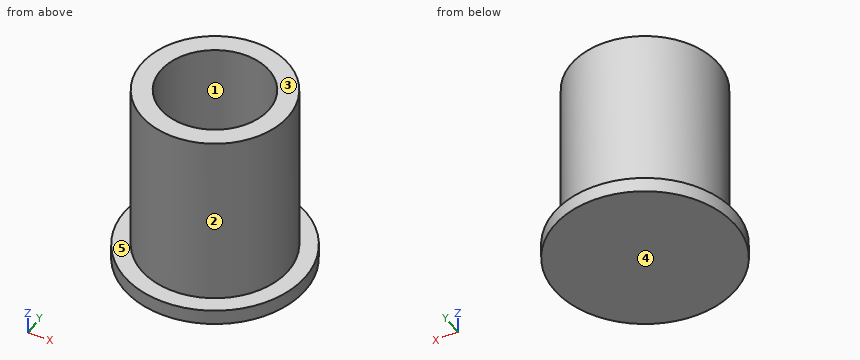
```python
from build123d import *

# Parameters (mm, degrees)
SKETCH_R     = 3
PAD_DEPTH    = 0.5
SKETCH001_R  = 2.435
PAD001_DEPTH = 5.8
SKETCH002_R  = 1.8
POCKET_DEPTH = 5.8


with BuildPart() as part:
    # Sketch (on Face1 of CopyBox) → Pad (new body)
    with BuildSketch(Plane.XY.offset(8)):
        Circle(SKETCH_R)
    extrude(amount=PAD_DEPTH)

    # Sketch001 (on Face3 of Pad) → Pad001 (join)
    with BuildSketch(Plane.XY.offset(8.5)):
        Circle(SKETCH001_R)
    extrude(amount=PAD001_DEPTH)

    # Sketch002 (on Face5 of Pad001) → Pocket (cut)
    with BuildSketch(Plane.XY.offset(14.3)):
        Circle(SKETCH002_R)
    extrude(amount=-POCKET_DEPTH, mode=Mode.SUBTRACT)


solid = part.part
```
Geometry check sheet. Reference: the model listing, model coordinates, mm. Face numbers are marked on the shaded views. A direction names the side the tool comes from. Round coordinates to 2 decimals unless told otherwise and drop trailing zeros. Loops run counter-clockwise (first coordinate to the right, second up) from the corner with the lowest first, then second, coordinate; pieces in that order, holes last. Notation, with made-up numbers: M -0.5,58.25 L 54.5,58.25 A19 cw 54.5,88.25 Z; hole C 5.5,60 d5. An arc over 180 degrees is marked long. Return JSON: item names as keys, results as strings. Group by question number.
(1) Scan lines: line 1 along Y through (x, z) = (0, 12.5) (3 decimals); line 2 along Z through (x, y) = (-1.25, -0.4); line 3 along X through (y, z) = (0.9, 11). Record each from-to range of solid material in increasing order. Write a range as [from, to].
(2) Section check B-B, the plane x = 0. Enter the section's corners in (y, z) (3 decimals).
(3) Section check D-D, the plane y = 2.35. Enter the section's corners in (x, z), and give its area (3 significant figures).
(4) Set-up check for the marked faces 4 and 5: record each of +Z, -Z, +X, -X, +Y, -Y from which the full face is reachable in a straight line by a thin tool's end or side.
(5) Section check A-A, the plane z = 11.25. Enter the section's corners in (x, y) (3 decimals).
(6) Mould release check, pull along X, two halves, no side actions. Record for the marked faces 1, 2 and 3: pulls with the +X half, pulls with the -X half, needs draft (parallel to the pull), parting line crosses it, or undercut.
(7) Go/stop test with flat-tipped pins: pin 1 (3 mm diameter, centred on y = 2, z = 10.5, fed in from +X); pin 2 (1.5 mm diameter, centred on x = -1, z = 13.5, fed in from -Y); pin 3 (1.8 mm diameter, centred on x = -0.5, y = -0.5, fed in from +Z). Record where each tip stops, or that it passes through.
Data:
{
 "1": {"line 1": "[-2.435, -1.8], [1.8, 2.435]", "line 2": "[8, 8.5]", "line 3": "[-2.26, -1.56], [1.56, 2.26]"},
 "2": {"outline": "M -3,8 L 3,8 L 3,8.5 L 2.435,8.5 L 2.435,14.3 L 1.8,14.3 L 1.8,8.5 L -1.8,8.5 L -1.8,14.3 L -2.435,14.3 L -2.435,8.5 L -3,8.5 Z"},
 "3": {"outline": "M -1.86,8 L 1.86,8 L 1.86,8.5 L 0.64,8.5 L 0.64,14.3 L -0.64,14.3 L -0.64,8.5 L -1.86,8.5 Z", "area": "9.26 mm²"},
 "4": {"face 4": "-Z, +X, -X, +Y, -Y", "face 5": "+Z"},
 "5": {"outline": "C 0,0 d4.87; hole C 0,0 d3.6"},
 "6": {"face 1": "undercut", "face 2": "parting line crosses it", "face 3": "needs draft"},
 "7": {"pin 1": "x = 2.38", "pin 2": "y = -2.42", "pin 3": "z = 8.5"}
}
